```python
from build123d import *

# Parameters (mm, degrees)
SKETCH_1_R          = 10
SKETCH_1_R_2        = 2.5
EXTRUDE_1_DEPTH     = 5
SKETCH_2_R          = 6
CUT_EXTRUDE_1_DEPTH = 1
SKETCH_3_R          = 0.9
CUT_EXTRUDE_2_DEPTH = 16


with BuildPart() as part:
    # 草图1 → 凸台-拉伸1 (new body)
    with BuildSketch(Plane(origin=(0, 0, 0), x_dir=(1, 0, 0), z_dir=(0, 1, 0))):
        with Locations(Location((0, 0, 0), (0, 0, 270))):
            Circle(SKETCH_1_R)
        with Locations(Location((0, 0, 0), (0, 0, 270))):
            Circle(SKETCH_1_R_2, mode=Mode.SUBTRACT)
    extrude(amount=EXTRUDE_1_DEPTH)

    # 草图2 → 切除-拉伸1 (cut)
    with BuildSketch(Plane(origin=(0, 5, 0), x_dir=(1, 0, 0), z_dir=(0, 1, 0))):
        with Locations(Location((0, 0, 0), (0, 0, 270))):
            Circle(SKETCH_2_R)
    extrude(amount=-CUT_EXTRUDE_1_DEPTH, mode=Mode.SUBTRACT)

    # 草图3 → 切除-拉伸2 (cut, through all)
    with BuildSketch(Plane(origin=(0, 5, 0), x_dir=(1, 0, 0), z_dir=(0, 1, 0))):
        with Locations(Location((0, 8, 0), (0, 0, 270))):
            Circle(SKETCH_3_R)
        with Locations(Location((8, 0, 0), (0, 0, 270))):
            Circle(SKETCH_3_R)
        with Locations(Location((0, -8, 0), (0, 0, 270))):
            Circle(SKETCH_3_R)
        with Locations(Location((-8, 0, 0), (0, 0, 270))):
            Circle(SKETCH_3_R)
    extrude(amount=-CUT_EXTRUDE_2_DEPTH, mode=Mode.SUBTRACT)


solid = part.part
```
Could you check a few things on this model? Use its own coordinates, in mm. A direction names the side the tool comes from. Round coordinates to 2 decimals unless told otherwise and drop trailing zeros. Loops run counter-clockwise (first coordinate to the right, second up) from the corner with the lowest first, then second, coordinate; pieces in that order, holes last. Notation, with made-up numbers: (19.5, 72.25) - (54.5, 72.25) arc R13 cw to (54.5, 83.25) - close; hole circle Ø3 at (27.25, 40). An arc over 180 degrees is marked (long way). Answer in a Markdown table with one row per item. Add a question column.
(1) I need wall thicknesses on line 1 along X through (y, z) = (3.45, -8); line 2 along X through (y, z) = (2.9, 0); line 3 along X through (y, z) = (4.4, 0). Which ranges of each line are inside material? Lowest first, please.
(2) If we section it at B-B (z = -8): Please give me the cut outline in (x, y).
(3) For faces 5 (the face through (0, 4, 3)), 6 (the face through (-7.11, 2.54, -0.12)), which set-ups out of +Z, -Z, +X, -X, +Y, -Y let a thin tool reach every point of the face, with its end or its side?
(4) If we section it at C-C (y = 0.35): Please give me the cut outline in (x, z).
(5) If we section it at D-D (x = -5.5): Please give me the cut outline in (y, z).
(6) If we section it at A-A (x = 8): Please give me the cut outline in (y, z), plus the area to 3 significant figures.
(7) If we mould it in two halves opening along Z, with no side actions, what happens to faces 1 (the face through (0, 2.5, -8.9)), 2 (the face through (-2, 0, 2)), 3 (the face through (1.802, 4.507, 5.723)), 4 (the face through (-9.76, 2.46, -2.17))? For each: pulls with the +Z half, pulls with the -Z half, needs draft (parallel to the pull), parting line crosses it, or undercut.
(8) I'm going to push flat-ended pins straight in: pin 1 (3.5 mm diameter, centred on x = -3, z = 1.5, fed in from +Y); pin 2 (2 mm diameter, centred on y = 3.5, z = -6, fed in from -X); pin 3 (1 mm diameter, centred on y = 2.5, z = -1.5, fed in from +X). Where does each tip first touch, or does it pass through?
Model answer:
| question | item | result |
|---|---|---|
| 1 | line 1 | x = -6 to -0.9, 0.9 to 6 |
| 1 | line 2 | x = -10 to -8.9, -7.1 to -2.5, 2.5 to 7.1, 8.9 to 10 |
| 1 | line 3 | x = -10 to -8.9, -7.1 to -6, 6 to 7.1, 8.9 to 10 |
| 2 | outline | (-6, 0) - (-0.9, 0) - (-0.9, 5) - (-6, 5) - close; (0.9, 0) - (6, 0) - (6, 5) - (0.9, 5) - close |
| 3 | face 5 | +Y |
| 3 | face 6 | +Y, -Y |
| 4 | outline | circle Ø20 at (0, 0); hole circle Ø1.8 at (-8, 0); hole circle Ø5 at (0, 0); hole circle Ø1.8 at (0, -8); hole circle Ø1.8 at (0, 8); hole circle Ø1.8 at (8, 0) |
| 5 | outline | (0, -8.35) - (5, -8.35) - (5, -2.4) - (4, -2.4) - (4, 2.4) - (5, 2.4) - (5, 8.35) - (0, 8.35) - close |
| 6 | outline | (0, -6) - (5, -6) - (5, -0.9) - (0, -0.9) - close; (0, 0.9) - (5, 0.9) - (5, 6) - (0, 6) - close |
| 6 | area | 51.0 mm² |
| 7 | face 1 | undercut |
| 7 | face 2 | needs draft |
| 7 | face 3 | undercut |
| 7 | face 4 | parting line crosses it |
| 8 | pin 1 | stops at y = 4 |
| 8 | pin 2 | stops at x = -8.66 |
| 8 | pin 3 | stops at x = 9.95 |
